The listing builds one solid part. Answer for the finished solid, in the listing's coordinates (mm). A direction names the side the tool comes from. Coordinates: 2 decimals unless noted, no trailing zeros. Loops run counter-clockwise (first coordinate to the right, second up) from the corner with the lowest first, then second, coordinate; pieces in that order, holes last. Notation, with made-up numbers: (59, 67.25) - (102, 67.25) arc R10 cw to (102, 79.25) - close; hole circle Ø9 at (-22.5, -15). An arc over 180 degrees is marked (long way). Return JSON: item names as keys, results as strings. Group by question number.
1. Section C-C (y = -24) is taken. Write down the section's boundary in (x, z), and give its area (3 significant figures).
2. Each of these flat-tipped pins is pushed along its axis until it touches: P1, Ø6.5, axis at x = 20.78, y = -12, coming from the -Z side; P2, Ø3, axis at x = 15, y = 18.5, coming from the +Z side; P3, Ø2, axis at y = -10, z = -14.5, coming from the -X side; P4, Ø0.8, axis at y = 9, z = -30.5, coming from the +X side. Where does it stop, or does it pass through?
3. Find the intervals of material crossed by line 1 along Y through (x, z) = (0, -1); line 2 along Y through (x, z) = (0, -35); line 3 along Z through (x, y) = (-21, -5.5), in increasing order.
4. The mould has two halves that part along Y. Classify faces 1 (the face through (2.5, 9, -21)), 2 (the face through (-6, 6, 0)), 3 (the face through (0, 10.3, -21)), 4 (the face through (16.128, -25.296, -3.042)): pulls with the +Y half, pulls with the -Y half, needs draft (parallel to the pull), parting line crosses it, or undercut.
5. Section D-D (z = -32.5) is taken. Write down the section's boundary in (x, y).
6. Section B-B (z = -2.5) is taken. Write down the section's boundary in (x, y), and give its area (3 significant figures).
7. Section A-A (x = 0) is taken. Write down the section's boundary in (y, z), and give its area (3 significant figures).
8. Which of the six approach directions +Z, -Z, +X, -X, +Y, -Y give full straight-line access (tool end or side, diameter ignored) to faces 5 (the face through (-3.47, 15.62, -24.73)), 6 (the face through (-2.5, 9, -21)), 7 (the face through (-3.8, -7.3, -41))?
```python
from build123d import *

# Parameters (mm, degrees)
CUT_EXTRUDE_1_REACH = 57
SKETCH_2_R          = 2.75
FILLET_1_R          = 2
SKETCH1_R           = 8
CUT_EXTRUDE1_DEPTH  = 60
CUT_EXTRUDE2_DEPTH  = 60


with BuildPart() as part:
    # 草图1 → 旋转1 (revolve)
    with BuildSketch(Plane(origin=(0, 0, 0), x_dir=(0, 0, -1), z_dir=(1, 0, 0)), mode=Mode.PRIVATE) as revolve_1_sk:
        Polygon((0, 0), (0, 30), (6, 30), (6, 16), (41, 16), (41, 0), align=None)
    revolve(revolve_1_sk.sketch.rotate(Axis((0, 0, 0), (0, 0, -1)), 90), axis=Axis((0, 0, 0), (0, 0, -1)))

    # 草图2 → 切除-拉伸1 (cut, up to next)
    with BuildSketch(Plane(origin=(0, 0, -6), x_dir=(-1, 0, 0), z_dir=(0, 0, -1)), mode=Mode.PRIVATE) as cut_extrude_1_sk1:
        with Locations((0, 24)):
            Circle(SKETCH_2_R)
    cut_extrude_1_tool1 = extrude(cut_extrude_1_sk1.sketch, amount=-CUT_EXTRUDE_1_REACH, mode=Mode.PRIVATE) & part.part
    # 草图2 → 切除-拉伸1 (cut, up to next)
    with BuildSketch(Plane(origin=(0, 0, -6), x_dir=(-1, 0, 0), z_dir=(0, 0, -1)), mode=Mode.PRIVATE) as cut_extrude_1_sk2:
        with Locations((20.784609691, 12)):
            Circle(SKETCH_2_R)
    cut_extrude_1_tool2 = extrude(cut_extrude_1_sk2.sketch, amount=-CUT_EXTRUDE_1_REACH, mode=Mode.PRIVATE) & part.part
    # 草图2 → 切除-拉伸1 (cut, up to next)
    with BuildSketch(Plane(origin=(0, 0, -6), x_dir=(-1, 0, 0), z_dir=(0, 0, -1)), mode=Mode.PRIVATE) as cut_extrude_1_sk3:
        with Locations((20.784609691, -12)):
            Circle(SKETCH_2_R)
    cut_extrude_1_tool3 = extrude(cut_extrude_1_sk3.sketch, amount=-CUT_EXTRUDE_1_REACH, mode=Mode.PRIVATE) & part.part
    # 草图2 → 切除-拉伸1 (cut, up to next)
    with BuildSketch(Plane(origin=(0, 0, -6), x_dir=(-1, 0, 0), z_dir=(0, 0, -1)), mode=Mode.PRIVATE) as cut_extrude_1_sk4:
        with Locations((0, -24)):
            Circle(SKETCH_2_R)
    cut_extrude_1_tool4 = extrude(cut_extrude_1_sk4.sketch, amount=-CUT_EXTRUDE_1_REACH, mode=Mode.PRIVATE) & part.part
    # 草图2 → 切除-拉伸1 (cut, up to next)
    with BuildSketch(Plane(origin=(0, 0, -6), x_dir=(-1, 0, 0), z_dir=(0, 0, -1)), mode=Mode.PRIVATE) as cut_extrude_1_sk5:
        with Locations((-20.784609691, -12)):
            Circle(SKETCH_2_R)
    cut_extrude_1_tool5 = extrude(cut_extrude_1_sk5.sketch, amount=-CUT_EXTRUDE_1_REACH, mode=Mode.PRIVATE) & part.part
    # 草图2 → 切除-拉伸1 (cut, up to next)
    with BuildSketch(Plane(origin=(0, 0, -6), x_dir=(-1, 0, 0), z_dir=(0, 0, -1)), mode=Mode.PRIVATE) as cut_extrude_1_sk6:
        with Locations((-20.784609691, 12)):
            Circle(SKETCH_2_R)
    cut_extrude_1_tool6 = extrude(cut_extrude_1_sk6.sketch, amount=-CUT_EXTRUDE_1_REACH, mode=Mode.PRIVATE) & part.part
    add(cut_extrude_1_tool1.solids().sort_by_distance((0, 24, -6))[0], mode=Mode.SUBTRACT)
    add(cut_extrude_1_tool2.solids().sort_by_distance((-20.78461, 12, -6))[0], mode=Mode.SUBTRACT)
    add(cut_extrude_1_tool3.solids().sort_by_distance((-20.78461, -12, -6))[0], mode=Mode.SUBTRACT)
    add(cut_extrude_1_tool4.solids().sort_by_distance((0, -24, -6))[0], mode=Mode.SUBTRACT)
    add(cut_extrude_1_tool5.solids().sort_by_distance((20.78461, -12, -6))[0], mode=Mode.SUBTRACT)
    add(cut_extrude_1_tool6.solids().sort_by_distance((20.78461, 12, -6))[0], mode=Mode.SUBTRACT)

    # 圆角1
    fillet_1_edges = [part.edges().sort_by_distance(p)[0] for p in [
        (-16, 0, -6),
    ]]
    fillet(fillet_1_edges, radius=FILLET_1_R)

    # Sketch1 → Cut-Extrude1 (cut, through all)
    with BuildSketch(Plane(origin=(0, 0, -41), x_dir=(-1, 0, 0), z_dir=(0, 0, -1))):
        Circle(SKETCH1_R)
    extrude(amount=-CUT_EXTRUDE1_DEPTH, mode=Mode.SUBTRACT)

    # Sketch2 → Cut-Extrude2 (cut, through all)
    with BuildSketch(Plane(origin=(0, 0, -41), x_dir=(-1, 0, 0), z_dir=(0, 0, -1))):
        with BuildLine():
            Line((-2.5, 7.599342077), (-2.5, 10.3))
            Line((-2.5, 10.3), (2.5, 10.3))
            Line((2.5, 10.3), (2.5, 7.599342077))
            ThreePointArc((2.5, 7.599342077), (0, 8), (-2.5, 7.599342077))
        make_face()
    extrude(amount=-CUT_EXTRUDE2_DEPTH, mode=Mode.SUBTRACT)


solid = part.part
```
The answers:
{
 "1": {"outline": "(-18, -6) - (-2.75, -6) - (-2.75, 0) - (-18, 0) - close; (2.75, -6) - (18, -6) - (18, 0) - (2.75, 0) - close", "area": "183 mm2"},
 "2": {"P1": "stops at z = -6", "P2": "stops at z = 0", "P3": "stops at x = -13.23", "P4": "stops at x = 13.49"},
 "3": {"line 1": "y = -30 to -26.75, -21.25 to -8, 10.3 to 21.25, 26.75 to 30", "line 2": "y = -16 to -8, 10.3 to 16", "line 3": "z = -6 to 0"},
 "4": {"face 1": "undercut", "face 2": "needs draft", "face 3": "undercut", "face 4": "parting line crosses it"},
 "5": {"outline": "circle Ø32 at (0, 0); hole (-2.5, 7.6) arc R8 ccw (long way) to (2.5, 7.6) - (2.5, 10.3) - (-2.5, 10.3) - close"},
 "6": {"outline": "circle Ø60 at (0, 0); hole circle Ø5.5 at (-20.78, -12); hole circle Ø5.5 at (-20.78, 12); hole circle Ø5.5 at (0, -24); hole circle Ø5.5 at (0, 24); hole (-2.5, 7.6) arc R8 ccw (long way) to (2.5, 7.6) - (2.5, 10.3) - (-2.5, 10.3) - close; hole circle Ø5.5 at (20.78, -12); hole circle Ø5.5 at (20.78, 12)", "area": "2,470 mm2"},
 "7": {"outline": "(-30, -6) - (-26.75, -6) - (-26.75, 0) - (-30, 0) - close; (-21.25, -6) - (-18, -6) arc R2 cw to (-16, -8) - (-16, -41) - (-8, -41) - (-8, 0) - (-21.25, 0) - close; (10.3, -41) - (16, -41) - (16, -8) arc R2 cw to (18, -6) - (21.25, -6) - (21.25, 0) - (10.3, 0) - close; (26.75, -6) - (30, -6) - (30, 0) - (26.75, 0) - close", "area": "665 mm2"},
 "8": {"face 5": "-Z", "face 6": "+Z, -Z", "face 7": "-Z, +X, -X, +Y, -Y"}
}
